```python
from build123d import *

# Parameters (mm, degrees)
F1_DEPTH = 25.4


with BuildPart() as f1:
    # F0 (on Top) → F1 (new body)
    with BuildSketch(Plane.XY):
        with BuildLine():
            Line((62.971446, 32.868891), (-38.628554, 32.868891))
            Line((-38.628554, 32.868891), (-38.628554, 16.993891))
            ThreePointArc((-38.628554, 16.993891), (-31.893362, 14.204083), (-29.103554, 7.468891))
            ThreePointArc((-29.103554, 7.468891), (-31.893362, 0.733699), (-38.628554, -2.056109))
            Line((-38.628554, -2.056109), (-38.628554, -17.931109))
            Line((-38.628554, -17.931109), (62.971446, -17.931109))
            Line((62.971446, -17.931109), (62.971446, 32.868891))
        make_face()
        with BuildLine():
            Line((-38.628554, 16.993891), (-38.628554, 32.868891))
            ThreePointArc((-38.628554, 32.868891), (-64.028554, 7.468891), (-38.628554, -17.931109))
            Line((-38.628554, -17.931109), (-38.628554, -2.056109))
            ThreePointArc((-38.628554, -2.056109), (-48.153554, 7.468891), (-38.628554, 16.993891))
        make_face()
    extrude(amount=F1_DEPTH)


solid = f1.part
```
Could you check a few things on this model? Use its own coordinates, in mm. Give positions to 0.01 mm unless a question says otherwise; leave off trailing zeros. Write each loop counter-clockwise with the first axis right and the second up, starting at its lowest first coordinate (ties: lowest second). Pieces come first, ordered by that corner, then holes. Notation, with made-up numbers: (19, -2.5) -> (61, -2.5) arc R18 cw to (61, 13.5) -> close; hole circle Ø9 at (43, 59.25). An arc over 180 degrees is marked (long way). Write each question's results on one line, items separated by ' | '.
1. Will this pin go through, and if not, where does the flat tip stop? pin 1 Ø1.5 at (y, z) = (3.5, 4.5) entering from -X.
Check sheet entries:
pin 1: stops at x = -63.82
2. I want a section at C-C, the plane x = -43. Write out the boundary of the cut face in (y, z).
Check sheet entries:
outline: (-17.55, 0) -> (-0.99, 0) -> (-0.99, 25.4) -> (-17.55, 25.4) -> close; (15.93, 0) -> (32.49, 0) -> (32.49, 25.4) -> (15.93, 25.4) -> close
3. I want a section at B-B, the plane y = 12. Write out the boundary of the cut face in (x, z), then the cut area to 3 significant figures.
Check sheet entries:
outline: (-63.62, 0) -> (-47.01, 0) -> (-47.01, 25.4) -> (-63.62, 25.4) -> close; (-30.25, 0) -> (62.97, 0) -> (62.97, 25.4) -> (-30.25, 25.4) -> close | area: 2,790 mm²
4. I want a section at D-D, the plane y = 23. Write out the boundary of the cut face in (x, z).
Check sheet entries:
outline: (-58.73, 0) -> (62.97, 0) -> (62.97, 25.4) -> (-58.73, 25.4) -> close
5. I need wall thicknesses on L1, parallel to X at y = 3, z = 9; L2, parallel to Y at x = -46.5, z = 21; L3, parallel to Y at x = -35, z = 18.75. Which ranges of each line are inside material? Lowest first, please.
Check sheet entries:
L1: x = -63.63 to -47.04, -30.22 to 62.97 | L2: y = -16.68 to 2.11, 12.83 to 31.62 | L3: y = -17.93 to -1.34, 16.28 to 32.87
6. I want a section at A-A, the plane z = 3.5. Write out the boundary of the cut face in (x, y) (3 decimals).
Check sheet entries:
outline: (-38.629, -17.931) -> (62.971, -17.931) -> (62.971, 32.869) -> (-38.629, 32.869) arc R25.4 ccw to start; hole circle Ø19.05 at (-38.629, 7.469)
